from build123d import *

# Parameters (mm, degrees)
F0_R     = 9
F1_DEPTH = 1.5
F2_R     = 9
F3_DEPTH = 1.5
F4_R     = 1
F5_R     = 3.1
F6_DEPTH = 7
F7_R     = 2
F9_DEPTH = 1.5


with BuildPart() as f1:
    # F0 (on Top) → F1 (new body)
    with BuildSketch(Plane.XY):
        Circle(F0_R)
        with BuildLine():
            add(Edge.make_bspline(
                [(0, 2.5), (-3.1781503931, 2.4996818975), (-6.0350862332, 1.3276056852), (-6, 0)],
                knots=[0, 0, 0, 0, 6.5, 6.5, 6.5, 6.5], degree=3))
            add(Edge.make_bspline(
                [(0, 2.5), (3.1781503931, 2.4996818975), (6.0350862332, 1.3276056852), (6, 0)],
                knots=[0, 0, 0, 0, 6.5, 6.5, 6.5, 6.5], degree=3))
            add(Edge.make_bspline(
                [(0, -2.5), (3.1781503931, -2.4996818975), (6.0350862332, -1.3276056852), (6, 0)],
                knots=[0, 0, 0, 0, 6.5, 6.5, 6.5, 6.5], degree=3))
            add(Edge.make_bspline(
                [(0, -2.5), (-3.1781503931, -2.4996818975), (-6.0350862332, -1.3276056852), (-6, 0)],
                knots=[0, 0, 0, 0, 6.5, 6.5, 6.5, 6.5], degree=3))
        make_face(mode=Mode.SUBTRACT)
    extrude(amount=F1_DEPTH)

    # F2 (on face) → F3 (join)
    with BuildSketch(Plane.XY.offset(1.5)):
        Circle(F2_R)
    extrude(amount=F3_DEPTH)

    # F4
    f4_edges = [f1.edges().sort_by_distance(p)[0] for p in [
        (-9, 0, 3),
    ]]
    fillet(f4_edges, radius=F4_R)

    # F5 (on face) → F6 (join)
    with BuildSketch(Plane.XY.offset(3)):
        Circle(F5_R)
    extrude(amount=F6_DEPTH)

    # F7
    f7_edges = [f1.edges().sort_by_distance(p)[0] for p in [
        (-3.1, 0, 10),
    ]]
    fillet(f7_edges, radius=F7_R)

    # F8 (on face) → F9 (join, through all)
    with BuildSketch(Plane(origin=(0, 0, 1.5), x_dir=(1, 0, 0), z_dir=(0, 0, -1))):
        with BuildLine():
            Line((0.5, 1.4), (0.5, 0))
            Line((0.5, 0), (0.5, -1.4))
            add(Edge.make_bspline(
                [(0.5, -1.4), (1.399901815, -1.3927484774), (2.9978926484, -1.1190434343), (3.9423397845, -0.7063065555)],
                knots=[0, 0, 0, 0, 2.9529043584, 2.9529043584, 2.9529043584, 2.9529043584], degree=3))
            ThreePointArc((3.9423397845, -0.7063065555), (3.7000016629, -0.0001318249), (3.94520464, 0.705053268))
            add(Edge.make_bspline(
                [(0.5, 1.4), (1.400812364, 1.39274114), (3.0011271582, 1.1184892747), (3.94520464, 0.705053268)],
                knots=[0, 0, 0, 0, 2.9558922002, 2.9558922002, 2.9558922002, 2.9558922002], degree=3))
        make_face()
        with BuildLine():
            Line((-0.5, 0), (-0.5, 1.4))
            add(Edge.make_bspline(
                [(-0.5, 1.4), (-1.400812364, 1.39274114), (-3.0011271582, 1.1184892747), (-3.94520464, 0.705053268)],
                knots=[0, 0, 0, 0, 2.9558922002, 2.9558922002, 2.9558922002, 2.9558922002], degree=3))
            ThreePointArc((-3.94520464, 0.705053268), (-3.7000016629, -0.0001318249), (-3.9423397845, -0.7063065555))
            add(Edge.make_bspline(
                [(-0.5, -1.4), (-1.399901815, -1.3927484774), (-2.9978926484, -1.1190434343), (-3.9423397845, -0.7063065555)],
                knots=[0, 0, 0, 0, 2.9529043584, 2.9529043584, 2.9529043584, 2.9529043584], degree=3))
            Line((-0.5, -1.4), (-0.5, 0))
        make_face()
    extrude(amount=F9_DEPTH)


solid = f1.part
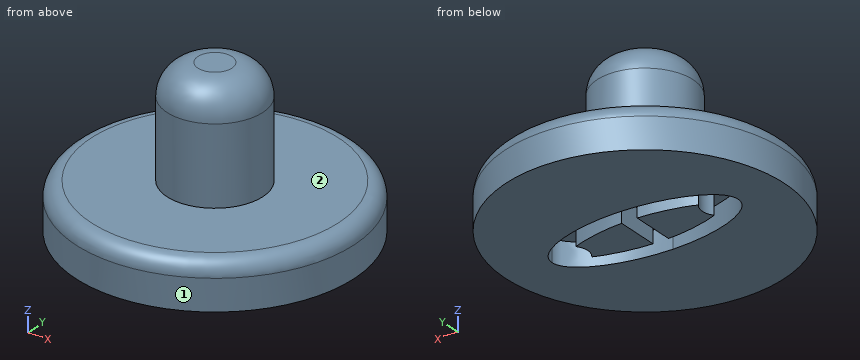
Geometry: final body of the model. Coordinates: model frame, mm. Face numbers are marked on the shaded views. A direction names the side the tool comes from. Give positions to 0.01 mm unless a question says otherwise; leave off trailing zeros. Loops run counter-clockwise (first coordinate to the right, second up) from the corner with the lowest first, then second, coordinate; pieces in that order, holes last. Notation, with made-up numbers: M 27,30.25 L 80,30.25 A34 ccw 80,64.25 Z; hole C 25,40 d11. An arc over 180 degrees is marked long. Put each result on its own line as item: value. Start each with the question number.
1) Ray query, line 1 along Z through (x, y) = (5, -4.5); line 2 along X through (y, z) = (2, 9.25); line 3 along X through (y, z) = (7, 2.75). Return the intervals inside material, ascending.
2) Cut plane A-A (z = 3.25). Output: boundary loops of the cut face in (x, y).
3) Contact query for a flat-ended pin moving along its axis: pin 1 (5 mm diameter, centred on y = 3, z = 2, fed in from +X). Output: stop coordinate, or through.
4) Access query for the marked faces 1 and 2. Directions: +Z, -Z, +X, -X, +Y, -Y. A direction counts if a zero-diameter tool reaches every point of the face in a straight line with its end or side. Return the directions, or none.
Verdict:
1. line 1: 0 to 3
1. line 2: -1.76 to 1.76
1. line 3: -5.1 to 5.1
2. outline: C 0,0 d6.2
3. pin 1: x = 8.99
4. face 1: +Z, -Z
4. face 2: +Z
